Autodesk Inventor part; units mm, degrees
ref_plane "YZ Plane" through (0, 0, 0) normal (1, 0, 0) x (0, 1, 0)
ref_plane "XZ Plane" through (0, 0, 0) normal (0, 1, 0) x (-1, 0, 0)
ref_plane "XY Plane" through (0, 0, 0) normal (0, 0, 1) x (1, 0, 0)
sketch "Sketch1" plane through (0, 0, 0) normal (0, 0, 1) x (1, 0, 0)
  circle A0 centre (31.0235, 53.7343) radius 2.5
  arc A1 (33.3294, 58.6976) -> (26.329, 56.4627) centre (30.8605, 54.3496) ccw
  arc A2 (20.0536, 53.8897) -> (26.329, 56.4627) centre (21.7974, 58.5758) ccw
  arc A3 (20.0536, 53.8897) -> (-20.0536, 53.8897) centre (0, 0) ccw
  arc A4 (-26.329, 56.4627) -> (-20.0536, 53.8897) centre (-21.7974, 58.5758) ccw
  arc A5 (-26.329, 56.4627) -> (-33.3294, 58.6976) centre (-30.8605, 54.3496) ccw
  arc A6 (-33.3294, 58.6976) -> (-34.1689, 58.2129) centre (0, 0) ccw
  arc A7 (-34.1689, 58.2129) -> (-35.7336, 51.0329) centre (-31.6379, 53.9008) ccw
  arc A8 (-36.643, 44.3118) -> (-35.7336, 51.0329) centre (-39.8294, 48.165) ccw
  arc A9 (-36.643, 44.3118) -> (-50.486, 27.5211) centre (0, 0) ccw
  line L0 (-50.486, 27.5211) -> (-42.3419, 27.5211)
  arc A10 (42.3419, 27.5211) -> (-42.3419, 27.5211) centre (0, 0) ccw
  line L1 (42.3419, 27.5211) -> (50.486, 27.5211)
  arc A11 (50.486, 27.5211) -> (36.643, 44.3118) centre (0, 0) ccw
  arc A12 (35.7336, 51.0329) -> (36.643, 44.3118) centre (39.8294, 48.165) ccw
  arc A13 (35.7336, 51.0329) -> (34.1689, 58.2129) centre (31.6379, 53.9008) ccw
  arc A14 (34.1689, 58.2129) -> (33.3294, 58.6976) centre (0, 0) ccw
  circle A15 centre (-31.0235, 53.7343) radius 2.5
  arc A16 (26.329, -56.4627) -> (33.3294, -58.6976) centre (30.8605, -54.3496) ccw
  arc A17 (33.3294, -58.6976) -> (34.1689, -58.2129) centre (0, 0) ccw
  arc A18 (34.1689, -58.2129) -> (35.7336, -51.0329) centre (31.6379, -53.9008) ccw
  arc A19 (36.643, -44.3118) -> (35.7336, -51.0329) centre (39.8294, -48.165) ccw
  arc A20 (36.643, -44.3118) -> (50.486, -27.5211) centre (0, 0) ccw
  line L2 (50.486, -27.5211) -> (42.3419, -27.5211)
  arc A21 (-42.3419, -27.5211) -> (42.3419, -27.5211) centre (0, 0) ccw
  line L3 (-42.3419, -27.5211) -> (-50.486, -27.5211)
  arc A22 (-50.486, -27.5211) -> (-36.643, -44.3118) centre (0, 0) ccw
  arc A23 (-35.7336, -51.0329) -> (-36.643, -44.3118) centre (-39.8294, -48.165) ccw
  arc A24 (-35.7336, -51.0329) -> (-34.1689, -58.2129) centre (-31.6379, -53.9008) ccw
  arc A25 (-34.1689, -58.2129) -> (-33.3294, -58.6976) centre (0, 0) ccw
  arc A26 (-33.3294, -58.6976) -> (-26.329, -56.4627) centre (-30.8605, -54.3496) ccw
  arc A27 (-20.0536, -53.8897) -> (-26.329, -56.4627) centre (-21.7974, -58.5758) ccw
  arc A28 (-20.0536, -53.8897) -> (20.0536, -53.8897) centre (0, 0) ccw
  arc A29 (26.329, -56.4627) -> (20.0536, -53.8897) centre (21.7974, -58.5758) ccw
  circle A30 centre (31.0235, -53.7343) radius 2.5
  circle A31 centre (-31.0235, -53.7343) radius 2.5
extrude "Extrusion1" add sketch "Sketch1" along normal blind 3.5
sketch "Sketch2" plane through (0, 0, 3.5) normal (0, 0, 1) x (1, 0, 0)
  circle A0 centre (-31.0235, 53.7343) radius 2.5
  circle A1 centre (31.0235, 53.7343) radius 2.5
  arc A2 (33.3294, 58.6976) -> (26.329, 56.4627) centre (30.8605, 54.3496) ccw
  arc A3 (20.0536, 53.8897) -> (26.329, 56.4627) centre (21.7974, 58.5758) ccw
  arc A4 (20.0536, 53.8897) -> (-20.0536, 53.8897) centre (0, 0) ccw
  arc A5 (-26.329, 56.4627) -> (-20.0536, 53.8897) centre (-21.7974, 58.5758) ccw
  arc A6 (-26.329, 56.4627) -> (-33.3294, 58.6976) centre (-30.8605, 54.3496) ccw
  arc A7 (-33.3294, 58.6976) -> (-34.1689, 58.2129) centre (0, 0) ccw
  arc A8 (-34.1689, 58.2129) -> (-35.7336, 51.0329) centre (-31.6379, 53.9008) ccw
  arc A9 (-36.643, 44.3118) -> (-35.7336, 51.0329) centre (-39.8294, 48.165) ccw
  arc A10 (-36.643, 44.3118) -> (-50.486, 27.5211) centre (0, 0) ccw
  line L0 (-50.486, 27.5211) -> (-42.3419, 27.5211)
  arc A11 (42.3419, 27.5211) -> (-42.3419, 27.5211) centre (0, 0) ccw
  line L1 (42.3419, 27.5211) -> (50.486, 27.5211)
  arc A12 (50.486, 27.5211) -> (36.643, 44.3118) centre (0, 0) ccw
  arc A13 (35.7336, 51.0329) -> (36.643, 44.3118) centre (39.8294, 48.165) ccw
  arc A14 (35.7336, 51.0329) -> (34.1689, 58.2129) centre (31.6379, 53.9008) ccw
  arc A15 (34.1689, 58.2129) -> (33.3294, 58.6976) centre (0, 0) ccw
  circle A16 centre (-31.0235, -53.7343) radius 2.5
  circle A17 centre (31.0235, -53.7343) radius 2.5
  arc A18 (26.329, -56.4627) -> (33.3294, -58.6976) centre (30.8605, -54.3496) ccw
  arc A19 (33.3294, -58.6976) -> (34.1689, -58.2129) centre (0, 0) ccw
  arc A20 (34.1689, -58.2129) -> (35.7336, -51.0329) centre (31.6379, -53.9008) ccw
  arc A21 (36.643, -44.3118) -> (35.7336, -51.0329) centre (39.8294, -48.165) ccw
  arc A22 (36.643, -44.3118) -> (50.486, -27.5211) centre (0, 0) ccw
  line L2 (50.486, -27.5211) -> (42.3419, -27.5211)
  arc A23 (-42.3419, -27.5211) -> (42.3419, -27.5211) centre (0, 0) ccw
  line L3 (-42.3419, -27.5211) -> (-50.486, -27.5211)
  arc A24 (-50.486, -27.5211) -> (-36.643, -44.3118) centre (0, 0) ccw
  arc A25 (-35.7336, -51.0329) -> (-36.643, -44.3118) centre (-39.8294, -48.165) ccw
  arc A26 (-35.7336, -51.0329) -> (-34.1689, -58.2129) centre (-31.6379, -53.9008) ccw
  arc A27 (-34.1689, -58.2129) -> (-33.3294, -58.6976) centre (0, 0) ccw
  arc A28 (-33.3294, -58.6976) -> (-26.329, -56.4627) centre (-30.8605, -54.3496) ccw
  arc A29 (-20.0536, -53.8897) -> (-26.329, -56.4627) centre (-21.7974, -58.5758) ccw
  arc A30 (-20.0536, -53.8897) -> (20.0536, -53.8897) centre (0, 0) ccw
  arc A31 (26.329, -56.4627) -> (20.0536, -53.8897) centre (21.7974, -58.5758) ccw
  arc A32 (-50.486, 27.5211) -> (-50.486, -27.5211) centre (0, 0) ccw
  arc A33 (50.486, -27.5211) -> (50.486, 27.5211) centre (0, 0) ccw
  line L4 (-18.0807, 31.3168) -> (-7.6035, 13.1696)
  arc A34 (-22.3885, 32.2819) -> (-39.1512, 3.248) centre (0, 0) ccw
  line L5 (-15.2069, 0) -> (-36.1615, 0)
  line L6 (-18.0807, -31.3168) -> (-7.6035, -13.1696)
  line L7 (7.6035, -13.1696) -> (18.0807, -31.3168)
  arc A35 (-16.7627, -35.53) -> (16.7627, -35.53) centre (0, 0) ccw
  line L8 (36.1615, 0) -> (15.2069, 0)
  line L9 (7.6035, 13.1696) -> (18.0807, 31.3168)
  arc A36 (39.1512, 3.248) -> (22.3885, 32.2819) centre (0, 0) ccw
  arc A37 (12.2636, 2.4194) -> (8.227, 9.4109) centre (0, 0) ccw
  arc A38 (-8.227, 9.4109) -> (-12.2636, 2.4194) centre (0, 0) ccw
  arc A39 (-4.0366, -11.8303) -> (4.0366, -11.8303) centre (0, 0) ccw
  arc A40 (-18.0807, 31.3168) -> (-22.3885, 32.2819) centre (-20.6788, 29.8168) ccw
  arc A41 (-39.1512, 3.248) -> (-36.1615, 0) centre (-36.1615, 3) ccw
  arc A42 (-15.2069, 0) -> (-12.2636, 2.4194) centre (-15.2069, 3) ccw
  arc A43 (-8.227, 9.4109) -> (-7.6035, 13.1696) centre (-10.2015, 11.6696) ccw
  spline S0 degree 3 poles (8.227, 9.4109) (8.2253, 9.4125) (8.2235, 9.414) (7.9828, 9.6254) (7.7777, 9.8729) (7.4513, 10.4284) (7.3317, 10.735) (7.19, 11.4166) (7.1804, 11.7904) (7.3007, 12.5134) (7.4219, 12.855) (7.6035, 13.1696) knots -0.433605 -0.433605 -0.433605 -0.433605 -0.432845 -0.432845 -0.329157 -0.329157 -0.224657 -0.224657 -0.109223 -0.109223 0 0 0 0
  arc A44 (22.3885, 32.2819) -> (18.0807, 31.3168) centre (20.6788, 29.8168) ccw
  arc A45 (36.1615, 0) -> (39.1512, 3.248) centre (36.1615, 3) ccw
  arc A46 (12.2636, 2.4194) -> (15.2069, 0) centre (15.2069, 3) ccw
  arc A47 (7.6035, -13.1696) -> (4.0366, -11.8303) centre (5.0054, -14.6696) ccw
  arc A48 (-4.0366, -11.8303) -> (-7.6035, -13.1696) centre (-5.0054, -14.6696) ccw
  arc A49 (-18.0807, -31.3168) -> (-16.7627, -35.53) centre (-15.4827, -32.8168) ccw
  arc A50 (16.7627, -35.53) -> (18.0807, -31.3168) centre (15.4827, -32.8168) ccw
  circle A51 centre (0, 0) radius 4.5
extrude "Extrusion2" add sketch "Sketch2" along normal blind 5
properties part number "bottom_shield"
For this review, take the finished solid that the model builds, in its own axes (mm). A direction names the side the tool comes from. Round coordinates to 2 decimals unless told otherwise and drop trailing zeros. Loops run counter-clockwise (first coordinate to the right, second up) from the corner with the lowest first, then second, coordinate; pieces in that order, holes last. Notation, with made-up numbers: (-37, 58.25) - (-4, 58.25) arc R32 ccw to (-4, 88.25) - close; hole circle Ø2 at (69, 25.5). An arc over 180 degrees is marked (long way). Use one line per item in the form item = value.
Item 1: Consider section B-B on y = 29.5. Write out the cut boundary in (x, z), then the cut area to 3 significant figures.
Answers:
outline = (-49.36, 0) - (-40.99, 0) - (-40.99, 3.5) - (-25.94, 3.5) - (-25.94, 8.5) - (-49.36, 8.5) - close; (-17.03, 3.5) - (17.03, 3.5) - (17.03, 8.5) - (-17.03, 8.5) - close; (25.94, 3.5) - (40.99, 3.5) - (40.99, 0) - (49.36, 0) - (49.36, 8.5) - (25.94, 8.5) - close
area = 463 mm^2
Item 2: Mouldability with a two-part tool opening along Y and no side actions: class faces 3 (the cylindrical face through (36.535, -54.909, 4.19)), 4 (the cylindrical face through (0.3, -57.5, 4.2)), 5 (the cylindrical face through (-23.65, 53.93, 4.19)) as +Y half, -Y half, draft (parallel to the pull), parting line (faces both ways), or undercut.
Answers:
face_3 = undercut
face_4 = -Y half
face_5 = +Y half
Item 3: Consider section A-A on x = 0. Write out the cut boundary in (y, z), then the cut area to 3 significant figures.
Answers:
outline = (-57.5, 0) - (-50.5, 0) - (-50.5, 3.5) - (-39.29, 3.5) - (-39.29, 8.5) - (-57.5, 8.5) - close; (-12.5, 3.5) - (-4.5, 3.5) - (-4.5, 8.5) - (-12.5, 8.5) - close; (4.5, 3.5) - (50.5, 3.5) - (50.5, 0) - (57.5, 0) - (57.5, 8.5) - (4.5, 8.5) - close
area = 445 mm^2
Item 4: Tool access review of faces 1 (the cylindrical face through (-57.5, -0.4, 6)), 2 (the cylindrical face through (6.03, -11.85, 5.96)): name each direction out of +Z, -Z, +X, -X, +Y, -Y from which nothing blocks a thin tool from reaching the whole face with its end or side.
Answers:
face_1 = +Z, -Z, -X
face_2 = +Z, -Z
Item 5: Clearance check with flat-ended pins moving along their axes: P1, Ø1, axis at x = -47, z = 1, coming from the +Y side; P2, Ø3, axis at y = -21.5, z = 1.5, coming from the +X side; P3, Ø1, axis at x = -47.5, z = 2.5, coming from the -Y side; P4, Ø6.5, axis at x = -31.02, y = -53.73, coming from the +Z side. State where each tip first meets the part, or that it passes through.
Answers:
P1 = 33.82
P2 = through
P3 = -33.12
P4 = 8.5
Item 6: For line 1 (X direction, y = -53.5, z = 8.25); line 2 (Y direction, x = 3, z = 7.75); line 3 (X direction, y = -0.5, z = 8.25), list the stretches that pass through material, from the lowest coordinate up.
Answers:
line_1 = -36.62 to -33.51, -28.53 to 28.53, 33.51 to 36.62
line_2 = -57.42 to -39.17, -12.13 to -3.35, 3.35 to 57.42
line_3 = -57.5 to -4.47, 4.47 to 57.5
Item 7: Consider section D-D on y = -20. Write out the cut boundary in (x, z), then the cut area to 3 significant figures.
Answers:
outline = (-53.91, 3.5) - (-11.55, 3.5) - (-11.55, 8.5) - (-53.91, 8.5) - close; (11.55, 3.5) - (53.91, 3.5) - (53.91, 8.5) - (11.55, 8.5) - close
area = 424 mm^2
Item 8: Consider section C-C on y = -33. Write out the cut boundary in (x, z).
Answers:
outline = (-47.09, 0) - (-38.23, 0) - (-38.23, 3.5) - (-18.48, 3.5) - (-18.48, 8.5) - (-47.09, 8.5) - close; (18.48, 3.5) - (38.23, 3.5) - (38.23, 0) - (47.09, 0) - (47.09, 8.5) - (18.48, 8.5) - close
